```python
from build123d import *

# Parameters (mm, degrees)
SKETCH1_W           = 177.8
SKETCH1_H           = 920.75
BOSS_EXTRUDE1_DEPTH = 12.7
CUT_EXTRUDE1_REACH  = 471.052
SKETCH2_W           = 101.6
SKETCH2_H           = 101.6


with BuildPart() as part:
    # Sketch1 → Boss-Extrude1 (new body)
    with BuildSketch(Plane.XY):
        Rectangle(SKETCH1_W, SKETCH1_H)
    extrude(amount=BOSS_EXTRUDE1_DEPTH)

    # Sketch2 → Cut-Extrude1 (cut, up to next)
    with BuildSketch(Plane(origin=(0, 0, 0), x_dir=(-1, 0, 0), z_dir=(0, 0, -1)), mode=Mode.PRIVATE) as cut_extrude1_sk1:
        with Locations((0, -365.125)):
            Rectangle(SKETCH2_W, SKETCH2_H)
    cut_extrude1_tool1 = extrude(cut_extrude1_sk1.sketch, amount=-CUT_EXTRUDE1_REACH, mode=Mode.PRIVATE) & part.part
    # Sketch2 → Cut-Extrude1 (cut, up to next)
    with BuildSketch(Plane(origin=(0, 0, 0), x_dir=(-1, 0, 0), z_dir=(0, 0, -1)), mode=Mode.PRIVATE) as cut_extrude1_sk2:
        with Locations((0, 384.875)):
            Rectangle(SKETCH2_W, SKETCH2_H)
    cut_extrude1_tool2 = extrude(cut_extrude1_sk2.sketch, amount=-CUT_EXTRUDE1_REACH, mode=Mode.PRIVATE) & part.part
    add(cut_extrude1_tool1.solids().sort_by_distance((0, -365.125, 0))[0], mode=Mode.SUBTRACT)
    add(cut_extrude1_tool2.solids().sort_by_distance((0, 384.875, 0))[0], mode=Mode.SUBTRACT)


solid = part.part
```
Verification items for the finished model (mm, model axes). Coordinates: 2 decimals unless noted, no trailing zeros. Loops run counter-clockwise (first coordinate to the right, second up) from the corner with the lowest first, then second, coordinate; pieces in that order, holes last. Notation, with made-up numbers: (88.5, 51) - (119.5, 51) arc R25 cw to (119.5, 69) - close; hole circle Ø6 at (58.25, 40). An arc over 180 degrees is marked (long way). Return JSON: item names as keys, results as strings.
1. Section check A-A, the plane x = 4. Record the boundary of the cut face in (y, z) (3 decimals), then the cut area to 3 significant figures.
Established:
{"outline": "(-460.375, 0) - (-415.925, 0) - (-415.925, 12.7) - (-460.375, 12.7) - close; (-314.325, 0) - (334.075, 0) - (334.075, 12.7) - (-314.325, 12.7) - close; (435.675, 0) - (460.375, 0) - (460.375, 12.7) - (435.675, 12.7) - close", "area": "9,110 mm2"}
2. Section check C-C, the plane z = 5. Record the boundary of the cut face in (x, y) (3 decimals).
Established:
{"outline": "(-88.9, -460.375) - (88.9, -460.375) - (88.9, 460.375) - (-88.9, 460.375) - close; hole (-50.8, -415.925) - (50.8, -415.925) - (50.8, -314.325) - (-50.8, -314.325) - close; hole (-50.8, 334.075) - (50.8, 334.075) - (50.8, 435.675) - (-50.8, 435.675) - close"}
3. Thickness scan on L1, parallel to Y at x = 50, z = 9.75 (3 decimals); L2, parallel to X at y = -333, z = 5.25. Record the ranges inside material, lowest first.
Established:
{"L1": "y = -460.375 to -415.925, -314.325 to 334.075, 435.675 to 460.375", "L2": "x = -88.9 to -50.8, 50.8 to 88.9"}
4. Section check B-B, the plane y = -324. Record the boundary of the cut face in (x, z).
Established:
{"outline": "(-88.9, 0) - (-50.8, 0) - (-50.8, 12.7) - (-88.9, 12.7) - close; (50.8, 0) - (88.9, 0) - (88.9, 12.7) - (50.8, 12.7) - close"}
